from build123d import *

# Parameters (mm, degrees)
BOSS_EXTRUDE1_DEPTH = 3
SKETCH2_R           = 2.15
CUT_EXTRUDE1_DEPTH  = 3


with BuildPart() as part:
    # Sketch1 → Boss-Extrude1 (new body)
    with BuildSketch(Plane.XY):
        Polygon((-352.325085215, 117.5), (-352.325085215, -117.5), (-337.325085215, -117.5), (-287.325085215, -67.5), (-287.325085215, 67.5), (-337.325085215, 117.5), align=None)
    extrude(amount=BOSS_EXTRUDE1_DEPTH)

    # Sketch2 → Cut-Extrude1 (cut)
    with BuildSketch(Plane(origin=(0, 0, 0), x_dir=(-1, 0, 0), z_dir=(0, 0, -1))):
        with Locations((344.825085215, 107.5)):
            Circle(SKETCH2_R)
        with Locations((344.825085215, 87.5)):
            Circle(SKETCH2_R)
        with Locations(Location((344.825085215, -87.5, 0), (0, 0, 180))):
            Circle(SKETCH2_R)
        with Locations(Location((344.825085215, -107.5, 0), (0, 0, 180))):
            Circle(SKETCH2_R)
        with Locations((297.325085215, 62.5)):
            Circle(SKETCH2_R)
        with Locations((307.325085215, 47.5)):
            Circle(SKETCH2_R)
        with Locations(Location((307.325085215, -47.5, 0), (0, 0, 180))):
            Circle(SKETCH2_R)
        with Locations(Location((297.325085215, -62.5, 0), (0, 0, 180))):
            Circle(SKETCH2_R)
    extrude(amount=-CUT_EXTRUDE1_DEPTH, mode=Mode.SUBTRACT)


solid = part.part
Verification items for the finished model (mm, model axes). Give positions to 0.01 mm unless a question says otherwise; leave off trailing zeros. Write each loop counter-clockwise with the first axis right and the second up, starting at its lowest first coordinate (ties: lowest second). Pieces come first, ordered by that corner, then holes.
(1) Material ranges on line 1 (X direction, y = -47.5, z = 1.05); line 2 (X direction, y = -107.5, z = 0.8); line 3 (Y direction, x = -329.5, z = 1.1), recorded low to high.
(2) Mould release check, pull along Y, two halves, no side actions. Record for faces 1 (the face through (-311.975, 92.15, 1.479)), 2 (the face through (-342.677, 87.595, 1.479)), 3 (the face through (-342.677, 107.595, 1.479)), 4 (the face through (-320, 2, 0)): +Y half, -Y half, draft (parallel to the pull), parting line (faces both ways), or undercut.
(3) Cross-section at A-A (y = 62.5). Enter the section's corners in (x, z).
(4) Cross-section at D-D (x = -322). Enter the section's corners in (y, z), plus the area to 3 significant figures.
(5) Gauge pin test, flat ends, axial feed: pin 1 (4 mm diameter, centred on x = -297.33, y = -62.5, fed in from +Z); pin 2 (3 mm diameter, centred on x = -335.5, y = 27, fed in from -Z). Record the tip position at first contact, or that the pin passes through.
(6) Cross-section at C-C (y = -87.5). Enter the section's corners in (x, z), plus the area to 3 significant figures.
(7) Cross-section at B-B (z = 2.55). State how many separate pieces and enclosed holes the cut face has, plus the area to 3 significant figures.
Worked out:
1. line 1: x = -352.33 to -309.48, -305.18 to -287.33
1. line 2: x = -352.33 to -346.98, -342.68 to -327.33
1. line 3: y = -109.67 to 109.67
2. face 1: +Y half
2. face 2: undercut
2. face 3: undercut
2. face 4: draft
3. outline: (-352.33, 0) - (-299.48, 0) - (-299.48, 3) - (-352.33, 3) - close; (-295.18, 0) - (-287.33, 0) - (-287.33, 3) - (-295.18, 3) - close
4. outline: (-102.17, 0) - (102.17, 0) - (102.17, 3) - (-102.17, 3) - close
4. area: 613 mm2
5. pin 1: passes through
5. pin 2: stops at z = 0
6. outline: (-352.33, 0) - (-346.98, 0) - (-346.98, 3) - (-352.33, 3) - close; (-342.68, 0) - (-307.33, 0) - (-307.33, 3) - (-342.68, 3) - close
6. area: 122 mm2
7. separate pieces: 1
7. enclosed holes: 8
7. area: 12,700 mm2
